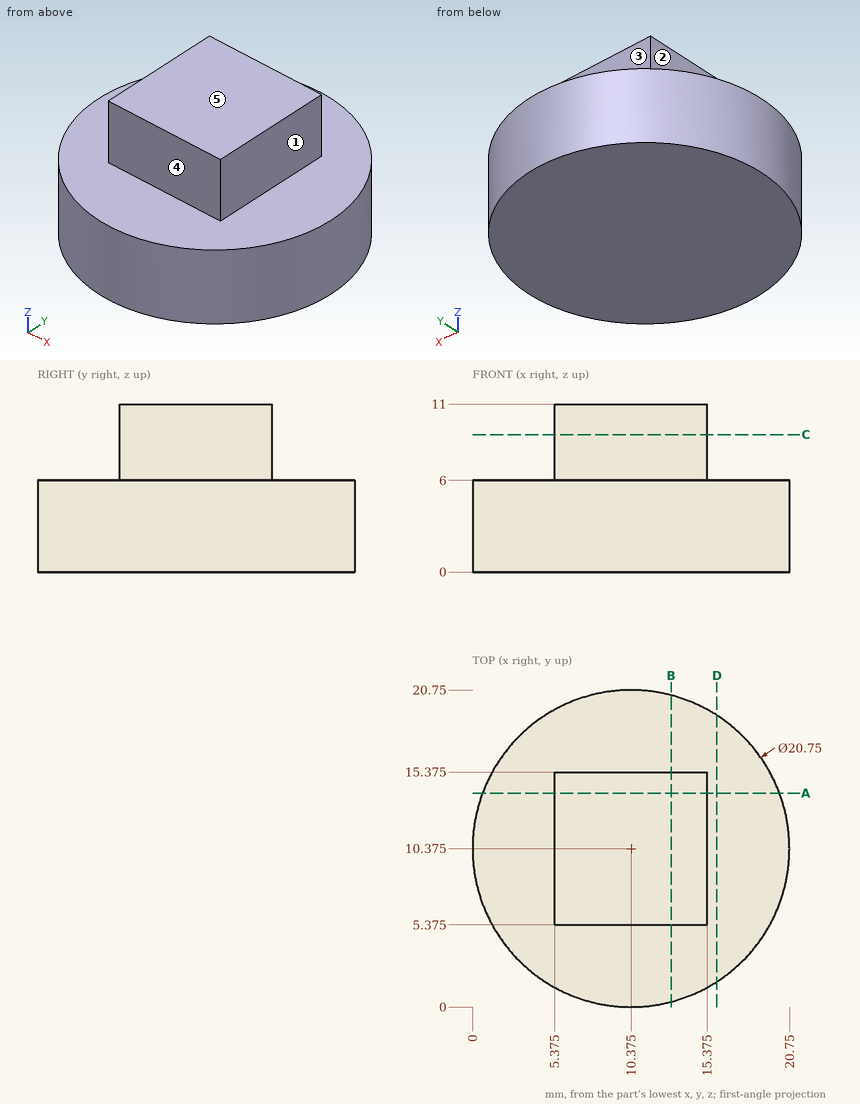
Job drawing, mm, ordinate dimensions from the low corner. One solid piece. A direction names the side the tool comes from. Round coordinates to 2 decimals unless told otherwise and drop trailing zeros. Write each loop counter-clockwise with the first axis right and the second up, starting at its lowest first coordinate (ties: lowest second). Pieces come first, ordered by that corner, then holes. Notation, with made-up numbers: (62.5, 72) -> (70.5, 72) arc R32 cw to (70.5, 104) -> close; hole circle Ø3 at (-15, -19.75). An arc over 180 degrees is marked (long way). Answer as CSV lines item,"result".
1. Slice it at D-D, the plane x = 16. List the corners of the cut face in (y, z), plus the area to 3 significant figures.
Resolved:
outline,"(1.66, 0) -> (19.09, 0) -> (19.09, 6) -> (1.66, 6) -> close"
area,"105 mm²"
2. Slice it at A-A, the plane y = 14. List the corners of the cut face in (x, z) (3 decimals).
Resolved:
outline,"(0.654, 0) -> (20.096, 0) -> (20.096, 6) -> (15.375, 6) -> (15.375, 11) -> (5.375, 11) -> (5.375, 6) -> (0.654, 6) -> close"
3. Slice it at C-C, the plane z = 9. List the corners of the cut face in (x, y) (3 decimals).
Resolved:
outline,"(5.375, 5.375) -> (15.375, 5.375) -> (15.375, 15.375) -> (5.375, 15.375) -> close"
4. Pin check, flat tips, straight feed: pin 1 Ø5.5 at (y, z) = (12, 9.5) entering from -X (3 decimals); pin 2 Ø1.5 at (x, z) = (9, 8) entering from +Y (3 decimals). Stop position of each tip, or through.
Resolved:
pin 1,"x = 5.375"
pin 2,"y = 15.375"
5. Tool access for the marked faces 1, 2, 3, 4 and 5: list every direction of +Z, -Z, +X, -X, +Y, -Y with a clear straight run to the whole face (end or side of a thin tool).
Resolved:
face 1,"+Z, +X, +Y, -Y"
face 2,"+Z, -X, +Y, -Y"
face 3,"+Z, +X, -X, +Y"
face 4,"+Z, +X, -X, -Y"
face 5,"+Z, +X, -X, +Y, -Y"
6. Slice it at B-B, the plane x = 13. List the corners of the cut face in (y, z) (3 decimals).
Resolved:
outline,"(0.338, 0) -> (20.412, 0) -> (20.412, 6) -> (15.375, 6) -> (15.375, 11) -> (5.375, 11) -> (5.375, 6) -> (0.338, 6) -> close"
7. Drill centre lines: line 1 (Y direction, x = 6.5, z = 8) (3 decimals); line 2 (Z direction, x = 7, y = 4). Where is each one in solid material? Low to high.
Resolved:
line 1,"5.375 to 15.375"
line 2,"0 to 6"
